from build123d import *

# Parameters (mm, degrees)
F2_R = 5
F3_R = 1.3428215566


with BuildPart() as f1:
    # F0 (on Front) → F1 (revolve)
    with BuildSketch(Plane.XZ):
        Polygon((-1.4891009778, 20.3513566048), (-1.4891009778, 8.119039867), (0, 9.0138781887), (0, 20.3513566048), align=None)
        Polygon((-1.4891009778, 8.119039867), (-15, 0), (0, 0), (0, 9.0138781887), align=None)
        Polygon((0, 0), (-15, 0), (-2.3833475581, -7.5784025668), (0, -9.01), align=None)
        Polygon((0, -9.01), (-2.3833475581, -7.5784025668), (0, -12.1514424682), align=None)
    revolve(axis=Axis((0, 0, -4.505), (0, 0, -1)))

    # F2
    f2_edges = [f1.edges().sort_by_distance(p)[0] for p in [
        (2.383348, 0, -7.578403),
    ]]
    fillet(f2_edges, radius=F2_R)

    # F3
    f3_edges = [f1.edges().sort_by_distance(p)[0] for p in [
        (1.489101, 0, 8.11904),
    ]]
    fillet(f3_edges, radius=F3_R)


solid = f1.part
Can you work these out from the model? Positions are in its coordinate system, mm. A direction names the side the tool comes from. Round coordinates to 2 decimals unless told otherwise and drop trailing zeros. Write each loop counter-clockwise with the first axis right and the second up, starting at its lowest first coordinate (ties: lowest second). Pieces come first, ordered by that corner, then holes. Notation, with made-up numbers: (6.25, 87) -> (14.25, 87) arc R29 ccw to (14.25, 114) -> close; hole circle Ø11 at (18, -17.5). An arc over 180 degrees is marked (long way). One line per question, with ' | ' between items. Start each with the question number.
1) On a 3-axis mill with a long thin cutter (end or side, diameter ignored), from which of +Z, -Z, +X, -X, +Y, -Y can I reach the whole of each face in a straight line? I mean faces 1 (the flat face through (0, 0, 20.351)), 2 (the cylindrical face through (-0.69, -1.32, 14.53)). Say none if no direction works.
2) Suppose I cut it at A-A on z = 17. Write out the boundary of the cut face in (x, y).
3) I need wall thicknesses on line 1 (Z direction, x = -5, y = -7.5); line 2 (Z direction, x = 12.5, y = 2); line 3 (X direction, y = 5.5, z = 2). Which ranges of each line are inside material? Lowest first, please. Write a range as [from, to].
4) I'm going to push flat-ended pins straight in: P1, Ø6, axis at x = -11, y = 10.5, coming from the +Z side; P2, Ø6, axis at x = -2, z = -3.5, coming from the -Y side; P3, Ø5, axis at x = 9, y = 0.5, coming from the -Z side. Where does each tip first touch, or does it pass through?
Return value:
1) face 1: +Z, +X, -X, +Y, -Y | face 2: +Z
2) outline: circle Ø2.98 at (0, 0)
3) line 1: z = [-3.6, 3.6] | line 2: z = [-1.41, 1.41] | line 3: x = [-10.29, 10.29]
4) P1: stops at z = 1.68 | P2: stops at y = -14.04 | P3: stops at z = -5.1
